Work out the finished part from the listing and answer in its coordinate system (mm). A direction names the side the tool comes from. Give positions to 0.01 mm unless a question says otherwise; leave off trailing zeros. Order: outer loops, then holes, each group sorted by start corner. A loop starts at its lowest first (then second) coordinate and runs counter-clockwise, first axis right, second up. Notation, with made-up numbers: (-22, 38) - (19, 38) arc R20 ccw to (19, 42) - close; hole circle Ø3 at (-36.5, -35.75). An arc over 180 degrees is marked (long way). Write each question's results on one line, items separated by ' | '.
from build123d import *

# Parameters (mm, degrees)
PAD_DEPTH = 10
FILLET_R  = 1


with BuildPart() as part:
    # Sketch → Pad (new body)
    with BuildSketch(Plane.XY):
        Polygon((0, 40), (-8.98056, 12.36068), (-38.042261, 12.36068), (-14.530851, -4.72136), (-23.51141, -32.36068), (0, -15), (23.51141, -32.36068), (14.530851, -4.72136), (38.042261, 12.36068), (8.98056, 12.36068), align=None)
    extrude(amount=PAD_DEPTH)

    # Fillet
    fillet_edges = [part.edges().sort_by_distance(p)[0] for p in [
        (38.042261, 12.36068, 5),
        (0, 40, 5),
        (-38.042261, 12.36068, 5),
        (-23.51141, -32.36068, 5),
        (23.51141, -32.36068, 5),
    ]]
    fillet(fillet_edges, radius=FILLET_R)


solid = part.part
1. A cutting plane is placed at A-A, the plane x = -15.5. Write down the section's boundary in (y, z).
Answer list:
outline: (-26.45, 0) - (-7.7, 0) - (-7.7, 10) - (-26.45, 10) - close; (-4.02, 0) - (12.36, 0) - (12.36, 10) - (-4.02, 10) - close
2. A cutting plane is placed at B-B, the plane z = 3.5. Write down the section's boundary in (x, y), then the cut area to 3 significant figures.
Answer list:
outline: (-35.55, 10.55) - (-14.53, -4.72) - (-22.55, -29.39) arc R1 ccw to (-21, -30.51) - (0, -15) - (21, -30.51) arc R1 ccw to (22.55, -29.39) - (14.53, -4.72) - (35.55, 10.55) arc R1 ccw to (34.96, 12.36) - (8.98, 12.36) - (0.95, 37.07) arc R1 ccw to (-0.95, 37.07) - (-8.98, 12.36) - (-34.96, 12.36) arc R1 ccw to start | area: 1,780 mm^2
3. Determine the mould class of faces 1 (the face through (-18.483, -16.885, 4.93)), 2 (the face through (22.2, -30.5, 5.1)), 3 (the face through (-1, 4, 10)) for opening direction X: +X half, -X half, draft (parallel to the pull), parting line (faces both ways), or undercut.
Answer list:
face 1: -X half | face 2: undercut | face 3: draft
4. Given P1, Ø12, axis at x = 1, y = -2.5, coming from the -Z side; P2, Ø3, axis at x = 13.5, z = 6.5, coming from the -Y side; P3, Ø1.5, axis at y = -13.5, z = 5.5, coming from the +X side; P4, Ø2, axis at x = 23, z = 9, coming from the -Y side, each flat-ended and moving along its own axis, determine where each tip first touches the part or whether it passes through.
Answer list:
P1: z = 0 | P2: y = -26.08 | P3: x = 17.63 | P4: y = -30.62
5. A cutting plane is placed at D-D, the plane x = 10. Write down the section's boundary in (y, z).
Answer list:
outline: (-22.38, 0) - (12.36, 0) - (12.36, 10) - (-22.38, 10) - close
6. Straight lines are drawn through the part: line 1 (X direction, y = -16, z = 3.25); line 2 (X direction, y = 32, z = 1.75); line 3 (Y direction, x = 24.5, z = 4). For each, find the intervals that lie inside material, in ascending order. Write a range as [from, to].
Answer list:
line 1: [-18.2, -1.35], [1.35, 18.2] | line 2: [-2.6, 2.6] | line 3: [2.52, 12.36]
7. A cutting plane is placed at C-C, the plane y = -20. Write down the section's boundary in (x, z), then the cut area to 3 significant figures.
Answer list:
outline: (-19.5, 0) - (-6.77, 0) - (-6.77, 10) - (-19.5, 10) - close; (6.77, 0) - (19.5, 0) - (19.5, 10) - (6.77, 10) - close | area: 254 mm^2
8. A tool of negligible diameter and unlimited length cuts with its end or side. For faces 4 (the face through (18.595, -17.231, 4.93)), 5 (the face through (-25.189, 3.022, 4.93)), 6 (the face through (-22, 12.361, 5)), 7 (the face through (22, 12.361, 5)), 8 (the face through (10.354, -22.646, 4.93)), from which of +Z, -Z, +X, -X, +Y, -Y can it reach the whole face along a straight path? Write none if from no direction.
Answer list:
face 4: +Z, -Z, +X | face 5: +Z, -Z, -X | face 6: +Z, -Z, -X, +Y | face 7: +Z, -Z, +X, +Y | face 8: +Z, -Z, -Y
